CAD build for the part. Positions are in the model's coordinates, mm. Face numbers are marked on the shaded views. A direction names the side the tool comes from. Give positions to 0.01 mm unless a question says otherwise; leave off trailing zeros. Write each loop counter-clockwise with the first axis right and the second up, starting at its lowest first coordinate (ties: lowest second). Pieces come first, ordered by that corner, then holes. Notation, with made-up numbers: (6, 85.25) - (40, 85.25) arc R10 ccw to (40, 97.25) - close; hole circle Ø4 at (84, 0). An arc over 180 degrees is marked (long way). Answer as a JSON object with one key per item and string values.
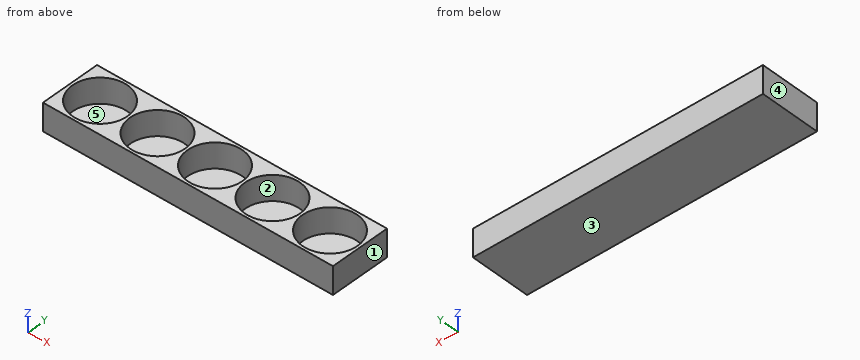
from build123d import *

# Parameters (mm, degrees)
F0_W     = 174
F0_H     = 36
F0_R     = 16.5
F1_DEPTH = 15
F2_W     = 174
F2_H     = 36
F3_DEPTH = 1.5


with BuildPart() as f1:
    # F0 (on Top) → F1 (new body)
    with BuildSketch(Plane.XY):
        with Locations((19.920273, 0)):
            Rectangle(F0_W, F0_H)
        with Locations((-49.079727, 0)):
            Circle(F0_R, mode=Mode.SUBTRACT)
        with Locations((-14.579727, 0)):
            Circle(F0_R, mode=Mode.SUBTRACT)
        with Locations((19.920273, 0)):
            Circle(F0_R, mode=Mode.SUBTRACT)
        with Locations((54.420273, 0)):
            Circle(F0_R, mode=Mode.SUBTRACT)
        with Locations((88.920273, 0)):
            Circle(F0_R, mode=Mode.SUBTRACT)
    extrude(amount=F1_DEPTH)

    # F2 (on face) → F3 (join)
    with BuildSketch(Plane(origin=(0, 0, 0), x_dir=(1, 0, 0), z_dir=(0, 0, -1))):
        with Locations((19.920273, 0)):
            Rectangle(F2_W, F2_H)
    extrude(amount=F3_DEPTH)


solid = f1.part
(1) 3-axis set-ups, long thin cutter, end or side, ignore diameter. For the marked faces 4 and 5: which of +Z, -Z, +X, -X, +Y, -Y reach the whole face in a straight line?
Answer key:
{"face 4": "+Z, -Z, -X, +Y, -Y", "face 5": "+Z"}
(2) Saw through at C-C, the plane x = -6. Give the cut face in (y, z).
Answer key:
{"outline": "(-18, -1.5) - (18, -1.5) - (18, 15) - (14.09, 15) - (14.09, 0) - (-14.09, 0) - (-14.09, 15) - (-18, 15) - close"}
(3) Pull direction X, two halves, no side cores. Call the marked faces 1, 2 and 3: pulls with the +X half, pulls with the -X half, needs draft (parallel to the pull), parting line crosses it, or undercut.
Answer key:
{"face 1": "pulls with the +X half", "face 2": "undercut", "face 3": "needs draft"}
(4) Probe L1, parallel to X at y = 1, z = 13.75; L2, parallel to Y at x = -14.5, z = 8; L3, parallel to X at y = -8, z = 10. List the from-to ranges inside material, lowest first. Write a range as [from, to].
Answer key:
{"L1": "x = [-67.08, -65.55], [-32.61, -31.05], [1.89, 3.45], [36.39, 37.95], [70.89, 72.45], [105.39, 106.92]", "L2": "y = [-18, -16.5], [16.5, 18]", "L3": "x = [-67.08, -63.51], [-34.65, -29.01], [-0.15, 5.49], [34.35, 39.99], [68.85, 74.49], [103.35, 106.92]"}
(5) Saw through at A-A, the plane y = 0. Give the cut face in (x, z).
Answer key:
{"outline": "(-67.08, -1.5) - (106.92, -1.5) - (106.92, 15) - (105.42, 15) - (105.42, 0) - (72.42, 0) - (72.42, 15) - (70.92, 15) - (70.92, 0) - (37.92, 0) - (37.92, 15) - (36.42, 15) - (36.42, 0) - (3.42, 0) - (3.42, 15) - (1.92, 15) - (1.92, 0) - (-31.08, 0) - (-31.08, 15) - (-32.58, 15) - (-32.58, 0) - (-65.58, 0) - (-65.58, 15) - (-67.08, 15) - close"}
(6) Saw through at B-B, the plane z = 5.25. Give the cut face in (x, y), and give its area (3 significant figures).
Answer key:
{"outline": "(-67.08, -18) - (106.92, -18) - (106.92, 18) - (-67.08, 18) - close; hole circle Ø33 at (-49.08, 0); hole circle Ø33 at (-14.58, 0); hole circle Ø33 at (19.92, 0); hole circle Ø33 at (54.42, 0); hole circle Ø33 at (88.92, 0)", "area": "1,990 mm²"}
(7) Flat gauge pin, fed straight in: P1, Ø2, axis at x = -8.5, y = -10.5, coming from the +Z side. Where does the tip first touch, or does it go through?
Answer key:
{"P1": "stops at z = 0"}
(8) Saw through at D-D, the plane y = -14.5. Give the cut face in (x, z), and give its area (3 significant figures).
Answer key:
{"outline": "(-67.08, -1.5) - (106.92, -1.5) - (106.92, 15) - (96.79, 15) - (96.79, 0) - (81.05, 0) - (81.05, 15) - (62.29, 15) - (62.29, 0) - (46.55, 0) - (46.55, 15) - (27.79, 15) - (27.79, 0) - (12.05, 0) - (12.05, 15) - (-6.71, 15) - (-6.71, 0) - (-22.45, 0) - (-22.45, 15) - (-41.21, 15) - (-41.21, 0) - (-56.95, 0) - (-56.95, 15) - (-67.08, 15) - close", "area": "1,690 mm²"}
